Answer from the drawing. Dimensions are ordinates in mm from the lowest x, y and z of the part. A direction names the side the tool comes from. Give positions to 0.01 mm unless a question says otherwise; leave off trailing zeros. Loops run counter-clockwise (first coordinate to the right, second up) from the corner with the lowest first, then second, coordinate; pieces in that order, holes last.
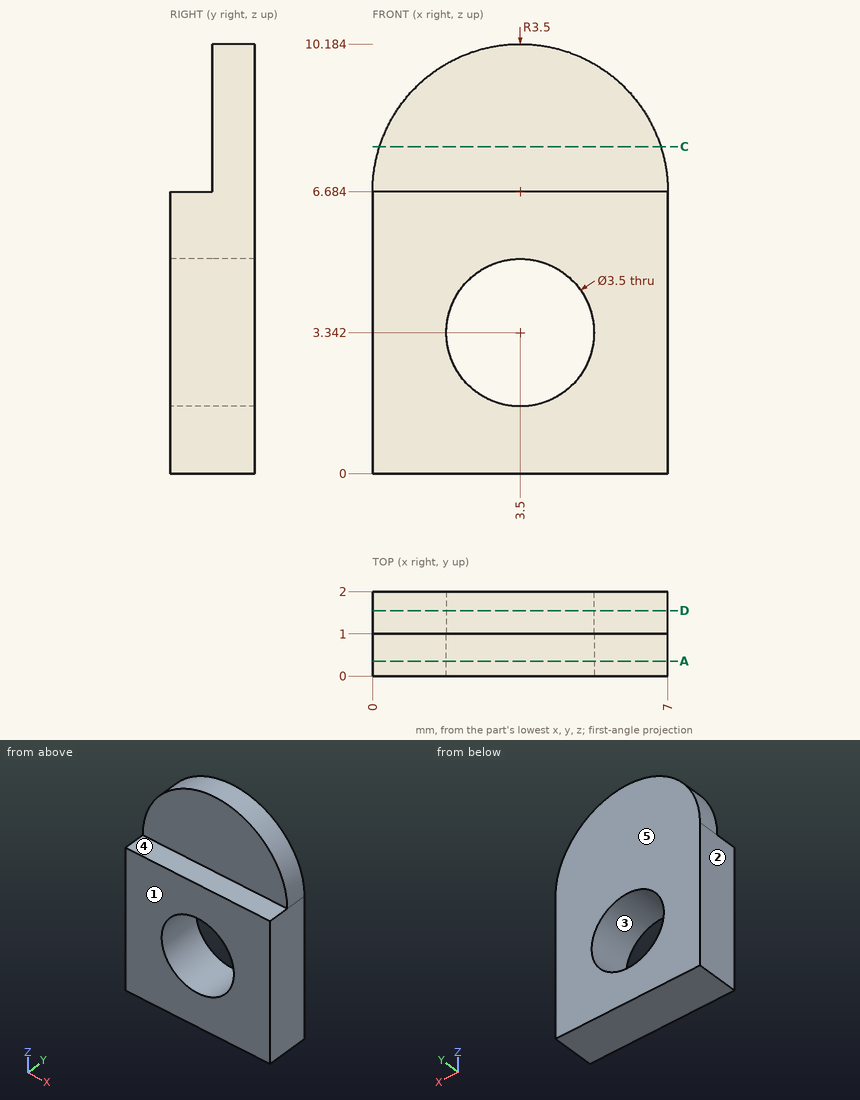
Item 1: Find section A-A, the plane y = 0.35. Write down the section's boundary in (x, z), plus the area to 3 significant figures.
Item 2: Find section C-C, the plane z = 7.75. Write down the section's boundary in (x, y), plus the area to 3 significant figures.
Item 3: Find section D-D, the plane y = 1.55. Write down the section's boundary in (x, z), plus the area to 3 significant figures.
Item 4: Determine the mould class of the marked faces 1, 2 and 3 for opening direction X: released by +X, released by -X, zero draft, split by the parting line, or undercut.
Item 5: Flat-ended cylindrical pins translate along their axes: pin 1 Ø0.8 at (x, y) = (3.5, 0.5) entering from +Z; pin 2 Ø3 at (x, z) = (3.5, 3.342) entering from +Y; pin 3 Ø1.1 at (x, z) = (4.5, 7.5) entering from -Y; pin 4 Ø2 at (x, z) = (4, 1.5) entering from -Y. Find the tip coordinate at first contact, or state that the pin passes through.
Item 6: For the marked faces 4 and 5, determine the directions among +Z, -Z, +X, -X, +Y, -Y from which every point of the face is accessible in a straight line to the end or side of a thin tool.
Item 7: Consider line 1 (Z direction, x = 3.5, y = 1.2); line 2 (Z direction, x = 3.5, y = 0.5); line 3 (Z direction, x = 1, y = 0.55). Determine where each line is inside the solid, lowest interval first.
Ans:
1. outline: (0, 0) - (7, 0) - (7, 6.68) - (0, 6.68) - close; hole circle Ø3.5 at (3.5, 3.34)
1. area: 37.2 mm2
2. outline: (0.17, 1) - (6.83, 1) - (6.83, 2) - (0.17, 2) - close
2. area: 6.67 mm2
3. outline: (0, 0) - (7, 0) - (7, 6.68) arc R3.5 ccw to (0, 6.68) - close; hole circle Ø3.5 at (3.5, 3.34)
3. area: 56.4 mm2
4. face 1: zero draft
4. face 2: released by -X
4. face 3: undercut
5. pin 1: stops at z = 6.68
5. pin 2: passes through
5. pin 3: stops at y = 1
5. pin 4: stops at y = 0
6. face 4: +Z, +X, -X, -Y
6. face 5: +Z, -Z, +X, -X, +Y
7. line 1: z = 0 to 1.59, 5.09 to 10.18
7. line 2: z = 0 to 1.59, 5.09 to 6.68
7. line 3: z = 0 to 6.68
